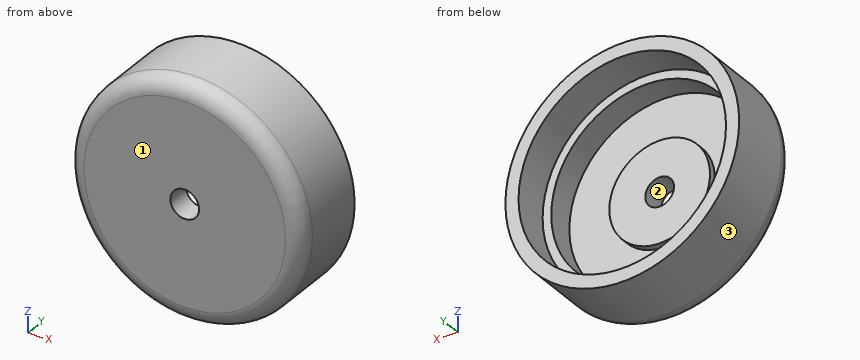
from build123d import *

# Parameters (mm, degrees)
FILLET1_R = 4.5


with BuildPart() as part:
    # Sketch2 → Revolve1 (revolve)
    with BuildSketch(Plane.XY):
        Polygon((4, 0), (28.52273273, 0), (32.5, 0), (32.5, 10), (32.5, 22), (28.85, 22), (28.85, 12), (26.45, 12), (26.45, 4.5), (14, 4.5), (14, 6.5), (4, 6.5), (4, 4), align=None)
    revolve(axis=Axis((0, 0, 0), (0, 1, 0)))

    # Fillet1
    fillet1_edges = [part.edges().sort_by_distance(p)[0] for p in [
        (-32.5, 0, 0),
    ]]
    fillet(fillet1_edges, radius=FILLET1_R)


solid = part.part
Source: CAD feature listing. Evaluate the final solid. Frame: model axes, mm. Face numbers are marked on the shaded views. Round coordinates to 2 decimals unless told otherwise and drop trailing zeros. Loops run counter-clockwise (first coordinate to the right, second up) from the corner with the lowest first, then second, coordinate; pieces in that order, holes last. Notation, with made-up numbers: M 3.25,8 L 39.25,8 A21 cw 39.25,33 Z; hole C 4.25,56 d4. An arc over 180 degrees is marked long. Return JSON: item names as keys, results as strings. Group by question number.
1. Section query B-B on z = 0. Output: boundary loops of the cut face in (x, y).
2. Pin query (flat end, axial travel): pin 1 (3 mm diameter, centred on x = 19.5, z = -18.5, fed in from -Y); pin 2 (8.5 mm diameter, centred on x = -5, z = 6.5, fed in from +Y); pin 3 (2 mm diameter, centred on x = 17, z = -17, fed in from +Y); pin 4 (1 mm diameter, centred on x = -22, y = 17.5, fed in from -Z). Return the tip coordinate at first contact, or that it passes through.
3. Material intervals for line 1 along Z through (x, y) = (-9.5, 6); line 2 along X through (y, z) = (7.25, 0); line 3 along X through (y, z) = (5.75, 4.5), sorted ascending. Write a range as from..to.
4. Section query D-D on y = 16. Output: boundary loops of the cut face in (x, z), and give its area (3 significant figures).
5. Section query C-C on y = 11. Output: boundary loops of the cut face in (x, z), and give its area (3 significant figures).
6. Section query A-A on x = 0. Output: boundary loops of the cut face in (y, z), and give its area (3 significant figures).
7. Mould query, pull axis X, two halves, no side actions, for the marked faces 1, 2 and 3. Classes: released by +X, released by -X, zero draft, split by the parting line, or undercut.
Checks:
{
 "1": {"outline": "M -32.5,4.5 A4.5 ccw -28,0 L -4,0 L -4,6.5 L -14,6.5 L -14,4.5 L -26.45,4.5 L -26.45,12 L -28.85,12 L -28.85,22 L -32.5,22 Z; M 4,0 L 28,0 A4.5 ccw 32.5,4.5 L 32.5,22 L 28.85,22 L 28.85,12 L 26.45,12 L 26.45,4.5 L 14,4.5 L 14,6.5 L 4,6.5 Z"},
 "2": {"pin 1": "stops at y = 0", "pin 2": "stops at y = 6.5", "pin 3": "stops at y = 4.5", "pin 4": "stops at z = -24.37"},
 "3": {"line 1": "z = -31.08..-24.69, -10.28..10.28, 24.69..31.08", "line 2": "x = -32.5..-26.45, 26.45..32.5", "line 3": "x = -32.19..-26.06, -13.26..13.26, 26.06..32.19"},
 "4": {"outline": "C 0,0 d65; hole C 0,0 d57.7", "area": "703 mm²"},
 "5": {"outline": "C 0,0 d65; hole C 0,0 d52.9", "area": "1,120 mm²"},
 "6": {"outline": "M 0,-28 A4.5 ccw 4.5,-32.5 L 22,-32.5 L 22,-28.85 L 12,-28.85 L 12,-26.45 L 4.5,-26.45 L 4.5,-14 L 6.5,-14 L 6.5,-4 L 0,-4 Z; M 0,4 L 6.5,4 L 6.5,14 L 4.5,14 L 4.5,26.45 L 12,26.45 L 12,28.85 L 22,28.85 L 22,32.5 L 4.5,32.5 A4.5 ccw 0,28 Z", "area": "452 mm²"},
 "7": {"face 1": "zero draft", "face 2": "undercut", "face 3": "split by the parting line"}
}
